from build123d import *

# Parameters (mm, degrees)
SKETCH1_W           = 254
SKETCH1_H           = 254
BOSS_EXTRUDE1_DEPTH = 5.08
SKETCH2_W           = 36.285714285
SKETCH2_H           = 5.08
SKETCH2_W_2         = 36.285714286
CUT_EXTRUDE1_DEPTH  = 5.08
SKETCH3_W           = 36.285714285
SKETCH3_H           = 5.08
SKETCH3_W_2         = 36.285714286
SKETCH3_W_3         = 37.524307816
CUT_EXTRUDE2_DEPTH  = 5.08
SKETCH4_W           = 36.285714285
SKETCH4_H           = 5.08
SKETCH4_W_2         = 36.285714286
CUT_EXTRUDE3_DEPTH  = 5.08
SKETCH5_W           = 36.285714285
SKETCH5_H           = 5.08
SKETCH5_W_2         = 36.285714286
CUT_EXTRUDE4_DEPTH  = 5.08
SKETCH6_W           = 29
SKETCH6_H           = 69
CUT_EXTRUDE5_DEPTH  = 5.08
CUT_EXTRUDE6_DEPTH  = 5.08
SKETCH8_W           = 5.08
SKETCH8_H           = 12.7
CUT_EXTRUDE7_DEPTH  = 5.08
SKETCH9_W           = 23
SKETCH9_H           = 5.08
CUT_EXTRUDE8_DEPTH  = 5.08
SKETCH10_W          = 23
SKETCH10_H          = 5.08
CUT_EXTRUDE9_DEPTH  = 5.08
SKETCH11_W          = 10.16
SKETCH11_H          = 6.35
CUT_EXTRUDE10_DEPTH = 5.08
SKETCH12_W          = 4.99581634
SKETCH12_H          = 3.489472518
CUT_EXTRUDE11_DEPTH = 5.08


with BuildPart() as part:
    # Sketch1 → Boss-Extrude1 (new body)
    with BuildSketch(Plane(origin=(0, 0, 0), x_dir=(1, 0, 0), z_dir=(0, 1, 0))):
        with Locations((-127, 127)):
            Rectangle(SKETCH1_W, SKETCH1_H)
    extrude(amount=BOSS_EXTRUDE1_DEPTH)

    # Sketch2 → Cut-Extrude1 (cut)
    with BuildSketch(Plane.XY):
        with Locations((-199.571428572, 2.54)):
            Rectangle(SKETCH2_W, SKETCH2_H)
        with Locations((-127, 2.54)):
            Rectangle(SKETCH2_W_2, SKETCH2_H)
        with Locations((-54.428571428, 2.54)):
            Rectangle(SKETCH2_W, SKETCH2_H)
    extrude(amount=-CUT_EXTRUDE1_DEPTH, mode=Mode.SUBTRACT)

    # Sketch3 → Cut-Extrude2 (cut)
    with BuildSketch(Plane(origin=(0, 0, 0), x_dir=(0, 0, -1), z_dir=(1, 0, 0))):
        with Locations((54.428571428, 2.54)):
            Rectangle(SKETCH3_W, SKETCH3_H)
        with Locations((127, 2.54)):
            Rectangle(SKETCH3_W_2, SKETCH3_H)
        with Locations((200.190725337, 2.54)):
            Rectangle(SKETCH3_W_3, SKETCH3_H)
    extrude(amount=-CUT_EXTRUDE2_DEPTH, mode=Mode.SUBTRACT)

    # Sketch4 → Cut-Extrude3 (cut)
    with BuildSketch(Plane(origin=(0, 0, -254), x_dir=(-1, 0, 0), z_dir=(0, 0, -1))):
        with Locations((54.428571428, 2.54)):
            Rectangle(SKETCH4_W, SKETCH4_H)
        with Locations((127, 2.54)):
            Rectangle(SKETCH4_W_2, SKETCH4_H)
        with Locations((199.571428572, 2.54)):
            Rectangle(SKETCH4_W, SKETCH4_H)
    extrude(amount=-CUT_EXTRUDE3_DEPTH, mode=Mode.SUBTRACT)

    # Sketch5 → Cut-Extrude4 (cut)
    with BuildSketch(Plane.ZY.offset(254)):
        with Locations((-199.571428572, 2.54)):
            Rectangle(SKETCH5_W, SKETCH5_H)
        with Locations((-127, 2.54)):
            Rectangle(SKETCH5_W_2, SKETCH5_H)
        with Locations((-54.428571428, 2.54)):
            Rectangle(SKETCH5_W, SKETCH5_H)
    extrude(amount=-CUT_EXTRUDE4_DEPTH, mode=Mode.SUBTRACT)

    # Sketch6 → Cut-Extrude5 (cut)
    with BuildSketch(Plane(origin=(0, 5.08, 0), x_dir=(1, 0, 0), z_dir=(0, 1, 0))):
        with Locations((-49, 204.26)):
            Rectangle(SKETCH6_W, SKETCH6_H)
        with Locations((-205, 204.26)):
            Rectangle(SKETCH6_W, SKETCH6_H)
    extrude(amount=-CUT_EXTRUDE5_DEPTH, mode=Mode.SUBTRACT)

    # Sketch7 → Cut-Extrude6 (cut)
    with BuildSketch(Plane(origin=(0, 5.08, 0), x_dir=(1, 0, 0), z_dir=(0, 1, 0))):
        Polygon((-51.54, 43.18), (-49, 43.18), (-46.46, 43.18), (-46.46, 55.88), (-51.54, 55.88), align=None)
    extrude(amount=-CUT_EXTRUDE6_DEPTH, mode=Mode.SUBTRACT)

    # Sketch8 → Cut-Extrude7 (cut)
    with BuildSketch(Plane(origin=(0, 5.08, 0), x_dir=(1, 0, 0), z_dir=(0, 1, 0))):
        with Locations((-205, 49.53)):
            Rectangle(SKETCH8_W, SKETCH8_H)
    extrude(amount=-CUT_EXTRUDE7_DEPTH, mode=Mode.SUBTRACT)

    # Sketch9 → Cut-Extrude8 (cut)
    with BuildSketch(Plane(origin=(-63.5, 0, 0), x_dir=(0, 0, -1), z_dir=(1, 0, 0))):
        with Locations((181.26, 2.54)):
            Rectangle(SKETCH9_W, SKETCH9_H)
        with Locations((227.26, 2.54)):
            Rectangle(SKETCH9_W, SKETCH9_H)
    extrude(amount=-CUT_EXTRUDE8_DEPTH, mode=Mode.SUBTRACT)

    # Sketch10 → Cut-Extrude9 (cut)
    with BuildSketch(Plane.ZY.offset(190.5)):
        with Locations((-181.26, 2.54)):
            Rectangle(SKETCH10_W, SKETCH10_H)
        with Locations((-227.26, 2.54)):
            Rectangle(SKETCH10_W, SKETCH10_H)
    extrude(amount=-CUT_EXTRUDE9_DEPTH, mode=Mode.SUBTRACT)

    # Sketch11 → Cut-Extrude10 (cut)
    with BuildSketch(Plane(origin=(0, 5.08, 0), x_dir=(1, 0, 0), z_dir=(0, 1, 0))):
        with Locations((-18.142857143, 18.142857143)):
            Rectangle(SKETCH11_W, SKETCH11_H)
    extrude(amount=-CUT_EXTRUDE10_DEPTH, mode=Mode.SUBTRACT)

    # Sketch12 → Cut-Extrude11 (cut)
    with BuildSketch(Plane(origin=(0, 5.08, 0), x_dir=(1, 0, 0), z_dir=(0, 1, 0))):
        with Locations((-235.857142857, 18.142857143)):
            Rectangle(SKETCH12_W, SKETCH12_H)
    extrude(amount=-CUT_EXTRUDE11_DEPTH, mode=Mode.SUBTRACT)


solid = part.part
Source: CAD feature listing. Evaluate the final solid. Frame: model axes, mm. Round coordinates to 2 decimals unless told otherwise and drop trailing zeros. Order: outer loops, then holes, each group sorted by start corner. A loop starts at its lowest first (then second) coordinate and runs counter-clockwise, first axis right, second up. Notation, with made-up numbers: (46.5, 65) - (68.5, 65) arc R35 cw to (68.5, 100) - close; hole circle Ø11 at (15.25, 46.5). An arc over 180 degrees is marked (long way). Use a Markdown table: item, result. Add a question column.
1. Line query: probe 1 along X at (y, z) = (3.5, -220.5); probe 2 along X at (y, z) = (1.4, -209); probe 3 along Z at (x, y) = (-15.5, 3.7). Output: solid intervals per line, ascending.
2. Section query D-D (x = -126.5). Return the cut outline in (y, z), then the cut area to 3 significant figures.
3. Section query B-B (z = -202). Return the cut outline in (x, y), then the cut area to 3 significant figures.
4. Section query C-C (y = 4). Give the number of separate pieces and of enclosed holes in the cut face, then the cut area to 3 significant figures.
5. First-contact query: pin 1 (1.5 mm diameter, centred on x = -18, y = 1.5, fed in from +Z); pin 2 (3 mm diameter, centred on x = -193.5, y = 1.5, fed in from +Z); pin 3 (2.5 mm diameter, centred on y = 3, z = -50.5, fed in from -X); pin 4 (2.5 mm diameter, centred on y = 3, z = -193, fed in from +X). Flat tips, straight axial feed; report the tip coordinate or a pass-through.
6. Section query A-A (x = -194). Return the cut outline in (y, z), then the cut area to 3 significant figures.
Derived:
| question | item | result |
|---|---|---|
| 1 | probe 1 | -254 to -219.5, -185.42 to -68.58, -34.5 to 0 |
| 1 | probe 2 | -248.92 to -219.5, -190.5 to -63.5, -34.5 to -5.08 |
| 1 | probe 3 | -254 to -21.32, -14.97 to 0 |
| 2 | outline | (0, -248.92) - (5.08, -248.92) - (5.08, -5.08) - (0, -5.08) - close |
| 2 | area | 1,240 mm2 |
| 3 | outline | (-248.92, 0) - (-219.5, 0) - (-219.5, 5.08) - (-248.92, 5.08) - close; (-190.5, 0) - (-63.5, 0) - (-63.5, 5.08) - (-190.5, 5.08) - close; (-34.5, 0) - (-5.08, 0) - (-5.08, 5.08) - (-34.5, 5.08) - close |
| 3 | area | 944 mm2 |
| 4 | separate pieces | 1 |
| 4 | enclosed holes | 6 |
| 4 | area | 57,600 mm2 |
| 5 | pin 1 | z = 0 |
| 5 | pin 2 | z = -5.08 |
| 5 | pin 3 | x = -248.92 |
| 5 | pin 4 | x = -5.08 |
| 6 | outline | (0, -248.92) - (5.08, -248.92) - (5.08, -238.76) - (0, -238.76) - close; (0, -169.76) - (5.08, -169.76) - (5.08, -5.08) - (0, -5.08) - close |
| 6 | area | 888 mm2 |
